Read the model definition and answer for the solid it produces. Units are mm, in the model's axes. Face numbers are marked on the shaded views. A direction names the side the tool comes from. Coordinates: 2 decimals unless noted, no trailing zeros. Write each loop counter-clockwise with the first axis right and the second up, starting at its lowest first coordinate (ties: lowest second). Pieces come first, ordered by that corner, then holes.
(1) Determine the mould class of the marked faces 1, 2 and 3 for opening direction X: pulls with the +X half, pulls with the -X half, needs draft (parallel to the pull), parting line crosses it, or undercut.
(2) The part is cut by section D-D, the plane z = -20.5. Determine the outline of the cut face in (x, y), and give its area (3 significant figures).
(3) The part is cut by section C-C, the plane x = -40.5. Determine the outline of the cut face in (y, z).
(4) Given pin 1 (17.5 mm diameter, centred on x = 21.5, z = 49.5, fed in from +Y); pin 2 (4 mm diameter, centred on x = -6.5, y = -19.5, fed in from +Z); pin 3 (2.5 mm diameter, centred on y = -2.5, z = -47, fed in from +X); pin 4 (12 mm diameter, centred on x = 1.5, y = -30, fed in from -Z), each flat-ended and moving along its own axis, determine where each tip first touches the part or whether it passes through.
(5) Which of the six approach directions +Z, -Z, +X, -X, +Y, -Y give full straight-line access (tool end or side, diameter ignored) to the marked faces 4 and 5?
(6) Straight lines are drawn through the part: line 1 along X through (y, z) = (-14, 0); line 2 along X through (y, z) = (-32.5, 0); line 3 along Y through (x, z) = (-17.5, 1). For each, find the intervals that lie inside material, in ascending order.
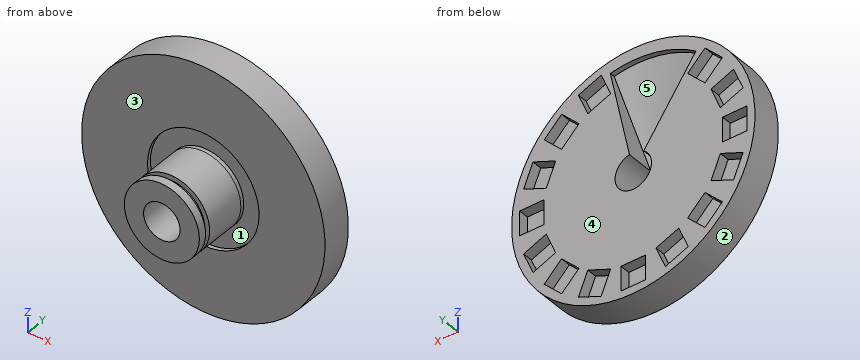
```python
from build123d import *

# Parameters (mm, degrees)
SKETCH3_W          = 12.15
SKETCH3_H          = 12.1
CUT_EXTRUDE1_DEPTH = 5
CIRPATTERN1_COUNT  = 16
CUT_SWEEP3_ANGLE   = 46.890766
SKETCH8_R          = 27.5
SKETCH8_R_2        = 18.5
CUT_EXTRUDE2_DEPTH = 1.85


# Read off the part's stored shape, not the designer's step: Cut-Sweep3
with BuildPart() as part:
    # Sketch1 → Revolve1 (revolve)
    with BuildSketch(Plane(origin=(0, 0, 0), x_dir=(0, 0, -1), z_dir=(1, 0, 0))):
        Polygon((9, 0), (60, 0), (60, -15), (18.5, -15), (18.5, -35), (16.100175422, -35), (16.100175422, -37.6), (18.5, -37.6), (18.5, -41.6), (9, -41.6), align=None)
    revolve(axis=Axis((0, 0, 0), (0, 1, 0)))

    # Sketch3 → Cut-Extrude1 (cut)
    with BuildSketch(Plane(origin=(0, 0, 0), x_dir=(1, 0, 0), z_dir=(0, 1, 0))):
        with Locations((0, 50)):
            Rectangle(SKETCH3_W, SKETCH3_H)
    cut_extrude1 = extrude(amount=-CUT_EXTRUDE1_DEPTH, mode=Mode.SUBTRACT)

    # CirPattern1: Cut-Extrude1 ×16 about axis, 2 skipped
    cirpattern1_axis = Axis((0, 0, 0), (0, -1, 0))
    add([cut_extrude1.rotate(cirpattern1_axis, i * 360 / CIRPATTERN1_COUNT) for i in range(1, CIRPATTERN1_COUNT) if i not in (8, 9)], mode=Mode.SUBTRACT)

    # Cut-Sweep3 outline → Cut-Sweep3 (revolve, cut)
    with BuildSketch(Plane(origin=(0, 0, 0), x_dir=(-0.5705578043075098, 0, 0.8212574455941287), z_dir=(-0.8212574455941287, 0, -0.5705578043075098))):
        Polygon((54.108249649, -2.5), (54.108249649, 0), (9, 0), (9, -13.715253714), align=None)
    revolve(axis=Axis((0, 0, 0), (0, 1, 0)), revolution_arc=CUT_SWEEP3_ANGLE, mode=Mode.SUBTRACT)

    # Sketch8 → Cut-Extrude2 (cut)
    with BuildSketch(Plane.XZ.offset(15)):
        with Locations(Location((0, 0, 0), (0, 0, 270))):
            Circle(SKETCH8_R)
        with Locations(Location((0, 0, 0), (0, 0, 270))):
            Circle(SKETCH8_R_2, mode=Mode.SUBTRACT)
    extrude(amount=-CUT_EXTRUDE2_DEPTH, mode=Mode.SUBTRACT)


solid = part.part
```
Computed:
1. face 1: undercut
1. face 2: parting line crosses it
1. face 3: needs draft
2. outline: (-56.39, -15) - (-18.33, -15) - (-18.33, -13.15) - (18.33, -13.15) - (18.33, -15) - (56.39, -15) - (56.39, 0) - (52.18, 0) - (52.18, -5) - (39.08, -5) - (39.08, 0) - (-39.08, 0) - (-39.08, -5) - (-52.18, -5) - (-52.18, 0) - (-56.39, 0) - close
2. area: 1,490 mm2
3. outline: (-15, -44.27) - (0, -44.27) - (0, -38.77) - (-5, -38.77) - (-5, -31.91) - (0, -31.91) - (0, -23.35) - (-5, -23.35) - (-5, -17.07) - (0, -17.07) - (0, 17.07) - (-5, 17.07) - (-5, 23.35) - (0, 23.35) - (0, 31.91) - (-5, 31.91) - (-5, 38.77) - (0, 38.77) - (0, 44.27) - (-15, 44.27) - close
4. pin 1: stops at y = 0
4. pin 2: stops at z = 17.94
4. pin 3: stops at x = 38.82
4. pin 4: stops at z = -18.5
5. face 4: +Z, -Z, +X, -X, +Y
5. face 5: +Y
6. line 1: x = -60 to -27.5, -18.5 to -9, 9 to 18.5, 27.5 to 60
6. line 2: x = -18.5 to -9, 9 to 18.5
6. line 3: y = -41.6 to -37.6, -35 to 0
